Geometry: final body of the model. Coordinates: model frame, mm. A direction names the side the tool comes from. Give positions to 0.01 mm unless a question says otherwise; leave off trailing zeros. Order: outer loops, then holes, each group sorted by start corner. A loop starts at its lowest first (then second) coordinate and runs counter-clockwise, first axis right, second up. Notation, with made-up numbers: (-26, 55) - (5, 55) arc R11 ccw to (5, 66) - close; hole circle Ø7 at (-29.5, 43.5). An arc over 180 degrees is marked (long way). One line per question, with ' | ' between items. Start each with the question number.
from build123d import *

# Parameters (mm, degrees)
SKETCH1_W           = 20
SKETCH1_H           = 40
BOSS_EXTRUDE1_DEPTH = 30
SKETCH2_W           = 40
SKETCH2_H           = 40
BOSS_EXTRUDE2_DEPTH = 20
FILLET1_R           = 10


with BuildPart() as part:
    # Sketch1 → Boss-Extrude1 (new body)
    with BuildSketch(Plane.XY):
        with Locations((-20, -20)):
            Rectangle(SKETCH1_W, SKETCH1_H)
    extrude(amount=BOSS_EXTRUDE1_DEPTH)

    # Sketch2 → Boss-Extrude2 (add)
    with BuildSketch(Plane.XY):
        with Locations((-10, -20)):
            Rectangle(SKETCH2_W, SKETCH2_H)
    extrude(amount=-BOSS_EXTRUDE2_DEPTH)

    # Fillet1
    fillet1_edges = [part.edges().sort_by_distance(p)[0] for p in [
        (0, 0, 0),
        (10, 0, -10),
        (-20, 0, 30),
    ]]
    fillet(fillet1_edges, radius=FILLET1_R)


solid = part.part
(1) Contact query for flat-ended pins moving along their axis: P1, Ø12, axis at x = 1.5, z = -2.5, coming from the +Y side; P2, Ø10, axis at x = -2.5, y = -27.5, coming from the +Z side; P3, Ø12, axis at y = -23.5, z = 18, coming from the +X side. Output: stop coordinate, or through.
(2) Cut plane A-A, the plane y = -15. Return the cut outline in (x, z), plus the area to 3 significant figures.
(3) Access query for faces 1 (the flat face through (0, -25, 0)), 2 (the flat face through (10, -25, -10)), 3 (the cylindrical face through (-2.08, -3.01, -2.85)). Directions: +Z, -Z, +X, -X, +Y, -Y. A direction counts if a zero-diameter tool reaches every point of the face in a straight line with its end or side. Return the directions, or none.
(4) Cut plane D-D, the plane y = -3. Return the cut outline in (x, z).
(5) Cut plane B-B, the plane z = -2. Return the cut outline in (x, y), plus the area to 3 significant figures.
(6) Cut plane C-C, the plane x = -7.5. Return the cut outline in (y, z).
(7) Material intervals for line 1 along X through (y, z) = (-14, 18); line 2 along Z through (x, y) = (-7.5, -32.5); line 3 along X through (y, z) = (-3.5, -8.5), sorted ascending. Write a range as from..to.
Results are:
1) P1: y = -0.11 | P2: z = 0 | P3: x = -10
2) outline: (-30, -20) - (10, -20) - (10, 0) - (-10, 0) - (-10, 30) - (-30, 30) - close | area: 1,400 mm2
3) face 1: +Z, +X, +Y, -Y | face 2: +Z, -Z, +X, +Y, -Y | face 3: +Z, +X, +Y
4) outline: (-30, -20) - (7.14, -20) - (7.14, -2.86) - (-10, -2.86) - (-10, 27.14) - (-30, 27.14) - close
5) outline: (-30, -40) - (10, -40) - (10, -10) arc R10 ccw to (8, -4) - (-10, -4) - (-10, 0) - (-30, 0) - close | area: 1,520 mm2
6) outline: (-40, -20) - (0, -20) - (0, -10) arc R10 ccw to (-10, 0) - (-40, 0) - close
7) line 1: -30..-10 | line 2: -20..0 | line 3: -30..7.6
